For this review, take the finished solid that the model builds, in its own axes (mm). Face numbers are marked on the shaded views. A direction names the side the tool comes from. Coordinates: 2 decimals unless noted, no trailing zeros. Loops run counter-clockwise (first coordinate to the right, second up) from the corner with the lowest first, then second, coordinate; pieces in that order, holes last. Notation, with made-up numbers: M 80.25,-1 L 100.25,-1 A7 cw 100.25,3 Z; hole C -17.5,-3 d1. An arc over 180 degrees is marked long. Write item = value, one per line.
from build123d import *

# Parameters (mm, degrees)
ESQUISSE1_W             = 59
ESQUISSE1_H             = 61
BOSS_EXTRU_1_DEPTH      = 35
COQUE1_T                = 2
CONG_1_R                = 1
ESQUISSE2_W             = 28.002662862
ESQUISSE2_H             = 31.996726322
ENL_V_MAT_EXTRU_1_DEPTH = 10
EMPREINTE1_START        = -31.5
EMPREINTE1_DEPTH        = 63
ENL_V_START             = -70
ENL_V_MAT_EXTRU_2_DEPTH = 70
ESQUISSE6_W             = 30.866772499
ESQUISSE6_H             = 33.57762677
BOSS_EXTRU_2_DEPTH      = 2
ESQUISSE5_W             = 26
ESQUISSE5_H             = 30
ENL_V_MAT_EXTRU_3_DEPTH = 12


# Read off the part's stored shape, not the designer's step: Empreinte1
with BuildPart() as part:
    # Esquisse1 → Boss.-Extru.1 (new body)
    with BuildSketch(Plane.XY):
        Rectangle(ESQUISSE1_W, ESQUISSE1_H)
    extrude(amount=BOSS_EXTRU_1_DEPTH)

    # Coque1
    coque1_openings = [part.faces().sort_by_distance(p)[0] for p in [
        (0, 0, 0),
    ]]
    offset(amount=COQUE1_T, openings=coque1_openings, kind=Kind.INTERSECTION)

    # Congé1
    # the kernel refuses this fillet: 1 mm, written as the material it takes off along each edge
    with BuildSketch(Plane(origin=(-31.5, 35, 37), x_dir=(0, 0, -1), z_dir=(0, -1, 0)), Plane(origin=(31.5, -35, 37), x_dir=(0, 0, -1), z_dir=(0, 1, 0))) as cong_1_piece_1:
        with BuildLine():
            CenterArc((CONG_1_R, CONG_1_R), CONG_1_R, 180, 90)
            Line((0, CONG_1_R), (0, 0))
            Line((0, 0), (CONG_1_R, 0))
        make_face()
    extrude(amount=70, mode=Mode.SUBTRACT)
    with BuildSketch(Plane(origin=(-34, -32.5, 37), x_dir=(0, 0, -1), z_dir=(1, 0, 0)), Plane(origin=(34, 32.5, 37), x_dir=(0, 0, -1), z_dir=(-1, 0, 0))) as cong_1_piece_2:
        with BuildLine():
            CenterArc((CONG_1_R, CONG_1_R), CONG_1_R, 180, 90)
            Line((0, CONG_1_R), (0, 0))
            Line((0, 0), (CONG_1_R, 0))
        make_face()
    extrude(amount=68, mode=Mode.SUBTRACT)

    # Esquisse2 → Enlèv. mat.-Extru.1 (cut)
    with BuildSketch(Plane.XY.offset(37)):
        with Locations((12.997811926, -9.999029903)):
            Rectangle(ESQUISSE2_W, ESQUISSE2_H)
    extrude(amount=-ENL_V_MAT_EXTRU_1_DEPTH, mode=Mode.SUBTRACT)

    # Empreinte1 outline → Empreinte1 (cut)
    with BuildSketch(Plane.YZ.offset(EMPREINTE1_START)):
        with BuildLine():
            Line((-32.5, 5.64631504), (-32.5, 2.461866011))
            ThreePointArc((-32.5, 2.461866011), (0.066578718, 7.992846788), (32.5, 1.728105633))
            Line((32.5, 1.728105633), (32.5, 4.938683524))
            ThreePointArc((32.5, 4.938683524), (0.062060176, 10.993081225), (-32.5, 5.64631504))
        make_face()
    extrude(amount=EMPREINTE1_DEPTH, mode=Mode.SUBTRACT)

    # Esquisse3 → Enlèv. mat.-Extru.2 (cut)
    with BuildSketch(Plane(origin=(31.5, 0, 0), x_dir=(0, 0, -1), z_dir=(1, 0, 0)).offset(ENL_V_START)):
        with BuildLine():
            Line((-1.728105633, 32.5), (0, 32.5))
            Line((0, 32.5), (0, -32.5))
            Line((0, -32.5), (-2.461866011, -32.5))
            ThreePointArc((-2.461866011, -32.5), (-7.992846788, 0.066578718), (-1.728105633, 32.5))
        make_face()
    extrude(amount=ENL_V_MAT_EXTRU_2_DEPTH, mode=Mode.SUBTRACT)

    # Esquisse6 → Boss.-Extru.2 (add)
    with BuildSketch(Plane.XY.offset(37)):
        with Locations((12.6560139, -10.131028325)):
            Rectangle(ESQUISSE6_W, ESQUISSE6_H)
    extrude(amount=-BOSS_EXTRU_2_DEPTH)

    # Esquisse5 → Enlèv. mat.-Extru.3 (cut)
    with BuildSketch(Plane.XY.offset(37)):
        with Locations((11.311132579, -9.001205365)):
            Rectangle(ESQUISSE5_W, ESQUISSE5_H)
    extrude(amount=-ENL_V_MAT_EXTRU_3_DEPTH, mode=Mode.SUBTRACT)


solid = part.part
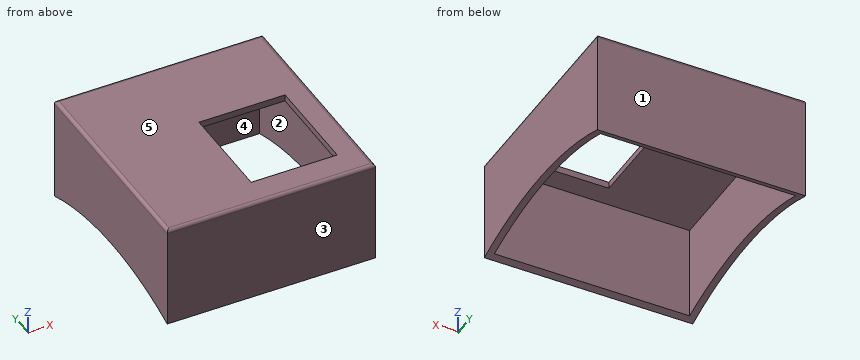
Q1. For line 1 along Y through (x, z) = (-21, 21.5); line 2 along X through (y, z) = (-20, 14.5); line 3 along Z through (x, y) = (-18.5, -3), list the stretches that pass through material, from the lowest coordinate up.
Solved:
line_1 = -32.5 to -30.5, 30.5 to 32.5
line_2 = -31.5 to -29.5, 29.5 to 31.5
line_3 = 35 to 37
Q2. For pin 1 Ø12 at (x, y) = (17, -25.5) entering from -Z; pin 2 Ø3 at (y, z) = (-11.5, 8.5) entering from -X; pin 3 Ø0.6 at (x, z) = (12, 36.5) entering from +Y, all flat-tipped, find the tip position at first contact; note any pin that passes through.
Solved:
pin_1 = 5.99
pin_2 = through
pin_3 = 32.48
Q3. Add section C-C (y = -5). Write out the cut boundary in (x, z), and give its area (3 significant figures).
Solved:
outline = M -31.5,10.91 L -29.5,10.91 L -29.5,35 L -1.69,35 L -1.69,37 L -30.5,37 A1 ccw -31.5,36 Z; M 24.31,35 L 29.5,35 L 29.5,10.91 L 31.5,10.91 L 31.5,36 A1 ccw 30.5,37 L 24.31,37 Z
area = 170 mm²
Q4. Machinability: for the marked faces 4 and 5, which of the approach directions +Z, -Z, +X, -X, +Y, -Y give a long, thin tool a straight path to every point of the face, cutting with its end or side? Answer none if there is none.
Solved:
face_4 = -Z
face_5 = +Z, +X, -X, +Y, -Y
Q5. Add section A-A (z = 24). Write out the cut boundary in (x, y), and give its area (3 significant figures).
Solved:
outline = M -31.5,-32.5 L 31.5,-32.5 L 31.5,32.5 L -31.5,32.5 Z; hole M -29.5,-30.5 L 29.5,-30.5 L 29.5,30.5 L -29.5,30.5 Z
area = 496 mm²
Q6. Add section B-B (x = 12). Write out the cut boundary in (y, z), and give its area (3 significant figures).
Solved:
outline = M -32.5,5.65 A95.5 cw -30.5,6.32 L -30.5,35 L -24,35 L -24,37 L -31.5,37 A1 ccw -32.5,36 Z; M 6,35 L 30.5,35 L 30.5,5.66 A95.5 cw 32.5,4.94 L 32.5,36 A1 ccw 31.5,37 L 6,37 Z
area = 187 mm²
Q7. Add section D-D (z = 7.5). Write out the cut boundary in (x, y), and give its area (3 significant figures).
Solved:
outline = M -31.5,-32.5 L 31.5,-32.5 L 31.5,-26.59 L 29.5,-26.59 L 29.5,-30.5 L -29.5,-30.5 L -29.5,-26.59 L -31.5,-26.59 Z; M -31.5,24.64 L -29.5,24.64 L -29.5,30.5 L 29.5,30.5 L 29.5,24.64 L 31.5,24.64 L 31.5,32.5 L -31.5,32.5 Z
area = 291 mm²
Q8. Draft analysis for pull direction Y (two halves, no side actions). For the marked faces 1, 2 and 3, state which applies: +Y half, -Y half, draft (parallel to the pull), parting line (faces both ways), or undercut.
Solved:
face_1 = +Y half
face_2 = undercut
face_3 = -Y half
